Check sheet for the modelled part. Datum: model origin and axes. Units: mm. Face numbers are marked on the shaded views. Give positions to 0.01 mm unless a question says otherwise; leave off trailing zeros. Write each loop counter-clockwise with the first axis right and the second up, starting at its lowest first coordinate (ties: lowest second). Pieces come first, ordered by that corner, then holes. Notation, with made-up numbers: M 88.25,66.25 L 131.25,66.25 A9 cw 131.25,76.25 Z; hole C 33,-8.5 d8. An arc over 180 degrees is marked long. One line per item, written item: value. Start each with the question number.
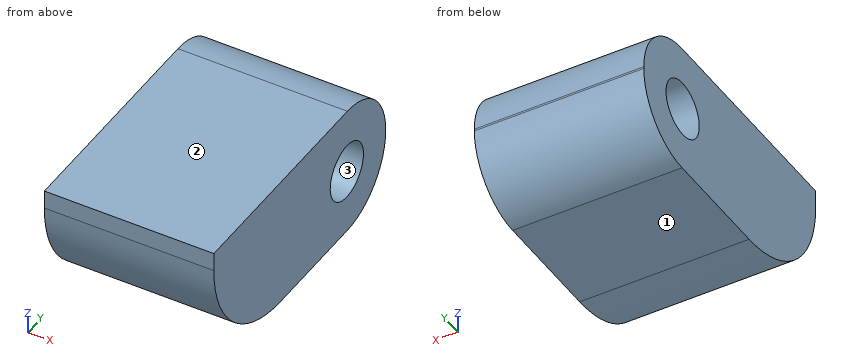
from build123d import *

# Parameters (mm, degrees)
CYLINDER002_R        = 1.5
CYLINDER002_DEPTH    = 11
BOX010_W             = 9
BOX010_H             = 15.5
BOX010_DEPTH         = 7
FILLET002008005010_R = 3.45
FILLET002008005011_R = 6


with BuildPart() as cylinder002:
    # Cylinder002 → Cylinder002 (new body)
    with BuildSketch(Plane(origin=(59, 25, 21.5), x_dir=(0, 0, -1), z_dir=(1, 0, 0))):
        Circle(CYLINDER002_R)
    extrude(amount=CYLINDER002_DEPTH)


with BuildPart() as cut:
    # Box010 → Box010 (new body)
    with BuildSketch(Plane(origin=(61, 13, 18), x_dir=(1, 0, 0), z_dir=(0, 0, 1))):
        with Locations((4.5, 7.75)):
            Rectangle(BOX010_W, BOX010_H)
    extrude(amount=BOX010_DEPTH)

    # Fillet002008005010
    fillet002008005010_edges = [cut.edges().sort_by_distance(p)[0] for p in [
        (65.5, 28.5, 18),
        (65.5, 28.5, 25),
    ]]
    fillet(fillet002008005010_edges, radius=FILLET002008005010_R)

    # Fillet002008005011
    fillet002008005011_edges = [cut.edges().sort_by_distance(p)[0] for p in [
        (65.5, 13, 18),
    ]]
    fillet(fillet002008005011_edges, radius=FILLET002008005011_R)

    # Cut: cut Cylinder002
    add(cylinder002.part, mode=Mode.SUBTRACT)


solid = cut.part
1) Cross-section at B-B (y = 24.5). Record the boundary of the cut face in (x, z), plus the area to 3 significant figures.
2) Draft check along Z on the marked faces 1, 2 and 3. Enter one of: released by +Z, released by -Z, zero draft, split by the parting line, or undercut.
3) Material ranges on L1, parallel to Z at x = 65.5, y = 25; L2, parallel to Y at x = 62.25, z = 21; L3, parallel to Y at x = 68, z = 21.5, recorded low to high. Write a range as from..to.
4) Cross-section at C-C (z = 19.5). Record the boundary of the cut face in (x, y), plus the area to 3 significant figures.
5) Cross-section at D-D (y = 15). Record the boundary of the cut face in (x, z), plus the area to 3 significant figures.
6) Cross-section at A-A (x = 64.5). Record the boundary of the cut face in (y, z), plus the area to 3 significant figures.
7) Gauge pin test, flat ends, axial feed: pin 1 (1.8 mm diameter, centred on y = 25, z = 21.5, fed in from +X); pin 2 (2 mm diameter, centred on x = 67, z = 21.5, fed in from -Y); pin 3 (1.5 mm diameter, centred on x = 62.5, z = 22.5, fed in from -Y). Record the tip position at first contact, or that the pin passes through.
Data:
1. outline: M 61,18 L 70,18 L 70,20.09 L 61,20.09 Z; M 61,22.91 L 70,22.91 L 70,25 L 61,25 Z
1. area: 37.5 mm2
2. face 1: released by -Z
2. face 2: released by +Z
2. face 3: undercut
3. L1: z = 18..20, 23..25
3. L2: y = 13.8..23.59, 26.41..28.47
3. L3: y = 13.55..23.5, 26.5..28.5
4. outline: M 61,15.03 L 70,15.03 L 70,27.9 L 61,27.9 Z
4. area: 116 mm2
5. outline: M 61,19.53 L 70,19.53 L 70,25 L 61,25 Z
5. area: 49.2 mm2
6. outline: M 13,24 A6 ccw 19,18 L 25.05,18 A3.45 ccw 28.5,21.45 L 28.5,21.55 A3.45 ccw 25.05,25 L 13,25 Z; hole C 25,21.5 d3
6. area: 88.6 mm2
7. pin 1: passes through
7. pin 2: stops at y = 13.19
7. pin 3: stops at y = 13.05
